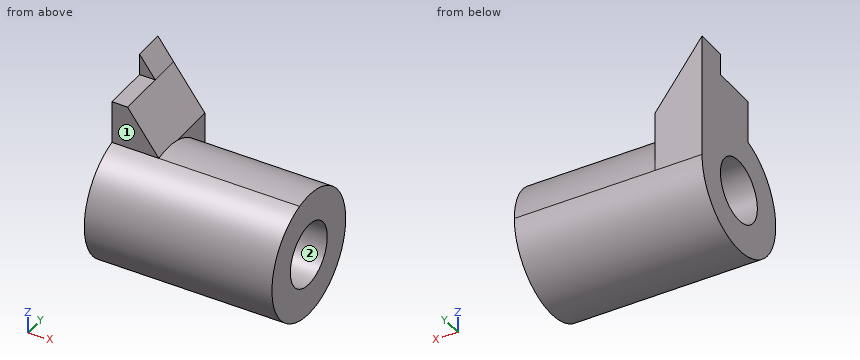
```python
from build123d import *

# Parameters (mm, degrees)
F0_W     = 76.2
F0_H     = 76.2
F1_DEPTH = 50.8
F2_R     = 12.7
F3_DEPTH = 76.201
F4_DEPTH = 57.15
F6_DEPTH = 31.751
F8_DEPTH = 12.701


with BuildPart() as f1:
    # F0 (on Front) → F1 (new body)
    with BuildSketch(Plane.XZ):
        with Locations((38.1, 38.1)):
            Rectangle(F0_W, F0_H)
    extrude(amount=F1_DEPTH)

    # F2 (on face) → F3 (cut, through all)
    with BuildSketch(Plane.YZ.offset(76.2)):
        with BuildLine():
            Line((-12.7, 67.4217641354), (-12.7, 76.2))
            Line((-12.7, 76.2), (-50.8, 76.2))
            Line((-50.8, 76.2), (-50.8, 25.4))
            ThreePointArc((-50.8, 25.4), (-45.4804631421, 40.9542598667), (-31.75, 49.9934442484))
            Line((-31.75, 49.9934442484), (-31.75, 67.4217641354))
            Line((-31.75, 67.4217641354), (-12.7, 67.4217641354))
        make_face()
        with BuildLine():
            Line((-50.8, 0), (-25.4, 0))
            ThreePointArc((-25.4, 0), (-43.3605122421, 7.4394877579), (-50.8, 25.4))
            Line((-50.8, 25.4), (-50.8, 0))
        make_face()
        with BuildLine():
            Line((0, 0), (0, 25.4))
            ThreePointArc((0, 25.4), (-7.4394877579, 7.4394877579), (-25.4, 0))
            Line((-25.4, 0), (0, 0))
        make_face()
        with Locations((-25.4, 25.4)):
            Circle(F2_R)
    extrude(amount=-F3_DEPTH, mode=Mode.SUBTRACT)

    # F2 (on face) → F4 (cut)
    with BuildSketch(Plane.YZ.offset(76.2)):
        with BuildLine():
            Line((0, 25.4), (0, 76.2))
            Line((0, 76.2), (-12.7, 76.2))
            Line((-12.7, 76.2), (-12.7, 67.4217641354))
            Line((-12.7, 67.4217641354), (-31.75, 67.4217641354))
            Line((-31.75, 67.4217641354), (-31.75, 49.9934442484))
            ThreePointArc((-31.75, 49.9934442484), (-9.8457401333, 45.4804631421), (0, 25.4))
        make_face()
    extrude(amount=-F4_DEPTH, mode=Mode.SUBTRACT)

    # F5 (on face) → F6 (cut, through all)
    with BuildSketch(Plane.XZ.offset(31.75)):
        Polygon((6.35, 67.4217641354), (19.05, 49.9934442484), (19.05, 67.4217641354), align=None)
    extrude(amount=-F6_DEPTH, mode=Mode.SUBTRACT)

    # F7 (on face) → F8 (cut, through all)
    with BuildSketch(Plane.XZ.offset(12.7)):
        Polygon((0, 76.2), (6.35, 67.4217641354), (19.05, 67.4217641354), (19.05, 76.2), align=None)
    extrude(amount=-F8_DEPTH, mode=Mode.SUBTRACT)


solid = f1.part
```
Can you work these out from the model? Positions are in its coordinate system, mm. Face numbers are marked on the shaded views. A direction names the side the tool comes from. Coordinates: 2 decimals unless noted, no trailing zeros. Loops run counter-clockwise (first coordinate to the right, second up) from the corner with the lowest first, then second, coordinate; pieces in that order, holes last. Notation, with made-up numbers: (77.25, 72) - (96.25, 72) arc R28 ccw to (96.25, 96) - close; hole circle Ø9 at (32.25, 87.25). An arc over 180 degrees is marked (long way). Answer as CSV lines item,"result". Start each with the question number.
1) Suppose I cut it at A-A (y = -25.4). Please give me the cut outline in (x, z), plus the area to 3 significant figures.
2) Which directions (+Z, -Z, +X, -X, +Y, -Y) give clear straight access to the entire face, cutting with the end or side of a thin tool? Please do the marked faces 1 and 2.
3) Suppose I cut it at D-D (y = -9). Please give me the cut outline in (x, z), plus the area to 3 significant figures.
4) I need wall thicknesses on line 1 (Z direction, x = 60, y = -25); line 2 (Y direction, x = 15, z = 25); line 3 (Y direction, x = 9, z = 52.5). Which ranges of each line are inside material? Lowest first, please. Write a range as from..to.
5) For pin 1 (3 mm diameter, centred on x = 48, z = 15, fed in from -Y); pin 2 (3 mm diameter, centred on x = 4.5, z = 71, fed in from -Y); pin 3 (3 mm diameter, centred on x = 16.5, z = 27.5, fed in from -Y); pin 4 (0.6 mm diameter, centred on y = -26, z = 50.5, fed in from -X), each with a flat end and sliding along its axis, tell me the tip position at first contact or that it passes through.
6) Suppose I cut it at C-C (z = 15.5). Please give me the cut outline in (x, y).
7) Suppose I cut it at B-B (x = 65). Please give me the cut outline in (y, z), plus the area to 3 significant figures.
Check result:
1,outline,"(0, 0) - (76.2, 0) - (76.2, 12.7) - (0, 12.7) - close; (0, 38.1) - (76.2, 38.1) - (76.2, 50.8) - (19.05, 50.8) - (19.05, 49.99) - (6.35, 67.42) - (0, 67.42) - close"
1,area,"2,140 mm²"
2,face 1,"+Z, +X, -X, -Y"
2,face 2,"+X, -X"
3,outline,"(0, 6) - (76.2, 6) - (76.2, 44.8) - (19.05, 44.8) - (19.05, 49.99) - (6.35, 67.42) - (0, 76.2) - close"
3,area,"3,300 mm²"
4,line 1,"z = 0..12.71, 38.09..50.8"
4,line 2,"y = -50.8..-38.09, -12.71..0"
4,line 3,"y = -31.75..0"
5,pin 1,"stops at y = -49.19"
5,pin 2,"stops at y = -12.7"
5,pin 3,"stops at y = -50.79"
5,pin 4,"stops at x = 0"
6,outline,"(0, -48.79) - (76.2, -48.79) - (76.2, -33.35) - (0, -33.35) - close; (0, -17.45) - (76.2, -17.45) - (76.2, -2.01) - (0, -2.01) - close"
7,outline,"circle Ø50.8 at (-25.4, 25.4); hole circle Ø25.4 at (-25.4, 25.4)"
7,area,"1,520 mm²"
